Check sheet for the drawn part. Datum: minimum x, y, z corner. Units: mm. A direction names the side the tool comes from. Coordinates: 2 decimals unless noted, no trailing zeros. Write each loop counter-clockwise with the first axis right and the second up, starting at its lowest first coordinate (ties: lowest second). Pieces come first, ordered by that corner, then holes. Notation, with made-up numbers: M 31,37.5 L 74,37.5 A21 ccw 74,47.5 Z; hole C 6.25,-2 d9. An arc over 180 degrees is marked long. Answer in a Markdown table with one row per item.
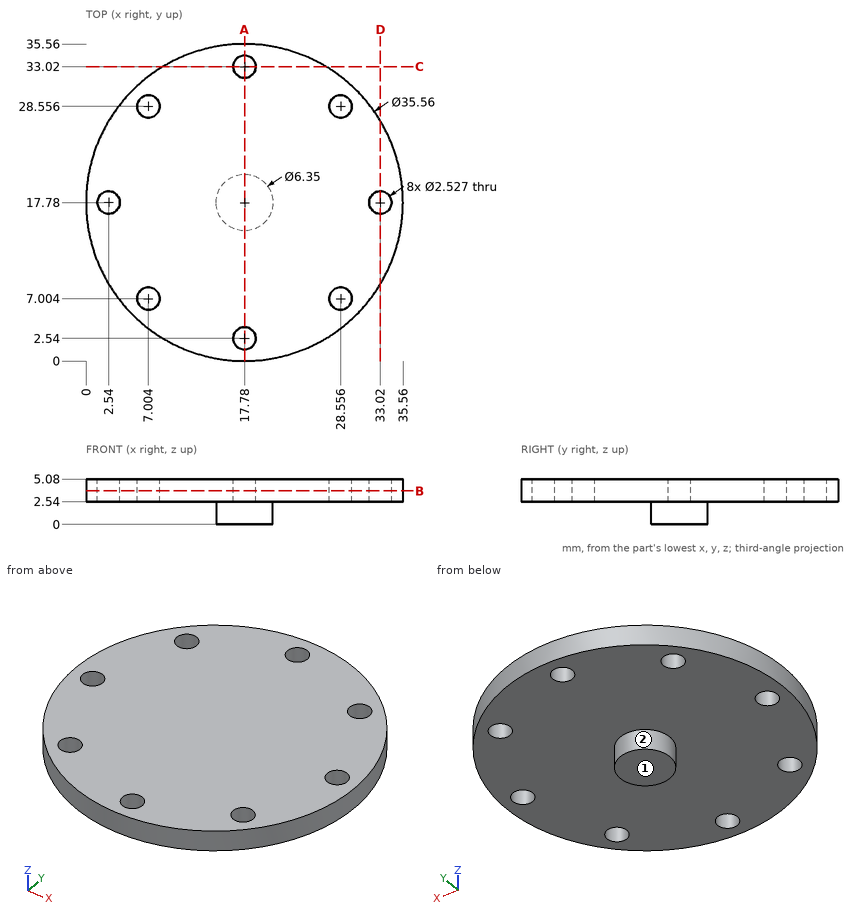
1) Depth check by flat-ended pin: pin 1 (1.5 mm diameter, centred on x = 2.54, y = 17.78, fed in from +Z); pin 2 (1.5 mm diameter, centred on x = 32, z = 4, fed in from -Y) (1 decimal); pin 3 (4 mm diameter, centred on x = 17.78, y = 33.02, fed in from -Z); pin 4 (1.5 mm diameter, centred on y = 25, z = 3.5, fed in from +X). Enter the tip coordinate at first touch or a pass-through.
Response values:
| item | result |
|---|---|
| pin 1 | passes through |
| pin 2 | stops at y = 6.2 |
| pin 3 | stops at z = 2.54 |
| pin 4 | stops at x = 34.34 |
2) Sectioned sample at A-A (x = 17.78). Record the cut outline in (y, z) (1 decimal).
Response values:
| item | result |
|---|---|
| outline | M 0,2.5 L 1.3,2.5 L 1.3,5.1 L 0,5.1 Z; M 3.8,2.5 L 14.6,2.5 L 14.6,0 L 21,0 L 21,2.5 L 31.8,2.5 L 31.8,5.1 L 3.8,5.1 Z; M 34.3,2.5 L 35.6,2.5 L 35.6,5.1 L 34.3,5.1 Z |
3) Sectioned sample at B-B (z = 3.75). Give the number of separate pieces and of enclosed holes in the cut face, then the cut area to 3 significant figures.
Response values:
| item | result |
|---|---|
| separate pieces | 1 |
| enclosed holes | 8 |
| area | 953 mm² |
4) Tool access check on the marked faces 1 and 2. Record the directions out of +Z, -Z, +X, -X, +Y, -Y that give a thin tool (end or side, any length) a straight path to the whole face; none if there is none.
Response values:
| item | result |
|---|---|
| face 1 | -Z, +X, -X, +Y, -Y |
| face 2 | -Z |
5) Thickness scan on L1, parallel to Y at x = 17.78, z = 3.6; L2, parallel to Z at x = 25.5, y = 10; L3, parallel to X at y = 2.54, z = 4 (1 decimal). Record the ranges inside material, lowest first. Write a range as [from, to].
Response values:
| item | result |
|---|---|
| L1 | y = [0, 1.28], [3.8, 31.76], [34.28, 35.56] |
| L2 | z = [2.54, 5.08] |
| L3 | x = [8.6, 16.5], [19, 26.9] |
6) Sectioned sample at C-C (y = 33.02). Record the cut outline in (x, z).
Response values:
| item | result |
|---|---|
| outline | M 8.62,2.54 L 16.52,2.54 L 16.52,5.08 L 8.62,5.08 Z; M 19.04,2.54 L 26.94,2.54 L 26.94,5.08 L 19.04,5.08 Z |
